Input: part model. Units: mm. Frame: model coordinates. Face numbers are marked on the shaded views. A direction names the side the tool comes from. Coordinates: 2 decimals unless noted, no trailing zeros. Order: outer loops, then holes, each group sorted by start corner. A loop starts at its lowest first (then second) coordinate and runs counter-clockwise, first axis right, second up. Notation, with made-up numbers: (5, 88) -> (51, 88) arc R8 ccw to (51, 95) -> close; hole circle Ø6 at (77, 84.25). An arc over 180 degrees is marked (long way). Answer as CSV lines item,"result".
from build123d import *

# Parameters (mm, degrees)
BOSS_EXTRUDE1_DEPTH      = 1.2
BOSS_EXTRUDE1_DEPTH_BACK = 1.2
SKETCH1_W                = 97
SKETCH1_H                = 71
SKETCH2_W                = 77
SKETCH2_H                = 51
CUT_EXTRUDE1_DEPTH       = 1.1
FILLET1_R                = 5
FILLET1_OF_MIRROR3_R     = 5
FILLET2_R                = 5


with BuildPart() as part:
    # Sketch1 → Boss-Extrude1 (new, two sides: drawn at the far end of the back side and taken through both)
    with BuildSketch(Plane(origin=(0, 0, 0), x_dir=(1, 0, 0), z_dir=(0, 1, 0)).offset(-BOSS_EXTRUDE1_DEPTH_BACK)):
        Rectangle(SKETCH1_W, SKETCH1_H)
    extrude(amount=BOSS_EXTRUDE1_DEPTH + BOSS_EXTRUDE1_DEPTH_BACK)

    # Sketch2 → Cut-Extrude1 (cut)
    with BuildSketch(Plane(origin=(0, 1.2, 0), x_dir=(1, 0, 0), z_dir=(0, 1, 0))):
        Rectangle(SKETCH2_W, SKETCH2_H)
    cut_extrude1 = extrude(amount=-CUT_EXTRUDE1_DEPTH, mode=Mode.SUBTRACT)

    # Fillet1
    fillet1_edges = [part.edges().sort_by_distance(p)[0] for p in [
        (38.5, 0.65, 25.5),
        (-38.5, 0.65, 25.5),
        (-38.5, 0.65, -25.5),
        (38.5, 0.65, -25.5),
    ]]
    fillet(fillet1_edges, radius=FILLET1_R)

    # Mirror3: Cut-Extrude1 across plane
    add(cut_extrude1.mirror(Plane.ZX), mode=Mode.SUBTRACT)

    # Fillet1 of Mirror3
    fillet1_of_mirror3_edges = [part.edges().sort_by_distance(p)[0] for p in [
        (38.5, -0.65, 25.5),
        (-38.5, -0.65, 25.5),
        (-38.5, -0.65, -25.5),
        (38.5, -0.65, -25.5),
    ]]
    fillet(fillet1_of_mirror3_edges, radius=FILLET1_OF_MIRROR3_R)

    # Fillet2
    fillet2_edges = [part.edges().sort_by_distance(p)[0] for p in [
        (48.5, 0, 35.5),
        (-48.5, 0, 35.5),
        (-48.5, 0, -35.5),
        (48.5, 0, -35.5),
    ]]
    fillet(fillet2_edges, radius=FILLET2_R)


solid = part.part
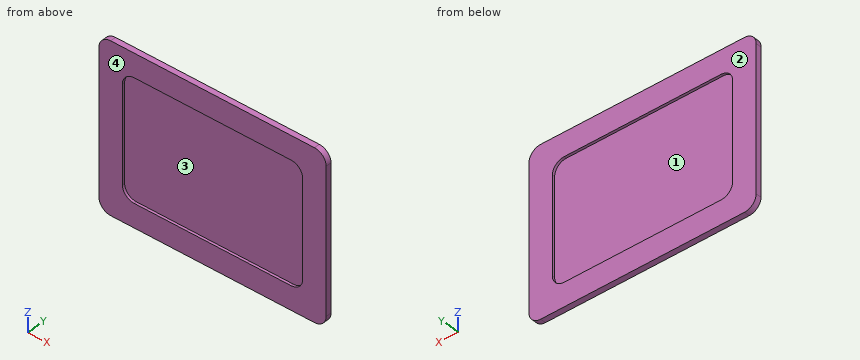
1. Cut plane A-A (y = -0.6). Return the cut outline in (x, z), plus the area to 3 significant figures.
Findings:
outline,"(-48.5, -30.5) arc R5 ccw to (-43.5, -35.5) -> (43.5, -35.5) arc R5 ccw to (48.5, -30.5) -> (48.5, 30.5) arc R5 ccw to (43.5, 35.5) -> (-43.5, 35.5) arc R5 ccw to (-48.5, 30.5) -> close; hole (-38.5, -20.5) arc R5 ccw to (-33.5, -25.5) -> (33.5, -25.5) arc R5 ccw to (38.5, -20.5) -> (38.5, 20.5) arc R5 ccw to (33.5, 25.5) -> (-33.5, 25.5) arc R5 ccw to (-38.5, 20.5) -> close"
area,"2,960 mm2"
2. Ray query, line 1 along X through (y, z) = (-1, 11); line 2 along Z through (x, y) = (-30.5, -0.6); line 3 along Y through (x, z) = (-35.5, -14.5). Return the intervals inside material, ascending.
Findings:
line 1,"x = -48.5 to -38.5, 38.5 to 48.5"
line 2,"z = -35.5 to -25.5, 25.5 to 35.5"
line 3,"y = -0.1 to 0.1"
3. Cut plane C-C (z = -7.5). Return the cut outline in (x, y).
Findings:
outline,"(-48.5, -1.2) -> (-38.5, -1.2) -> (-38.5, -0.1) -> (38.5, -0.1) -> (38.5, -1.2) -> (48.5, -1.2) -> (48.5, 1.2) -> (38.5, 1.2) -> (38.5, 0.1) -> (-38.5, 0.1) -> (-38.5, 1.2) -> (-48.5, 1.2) -> close"
4. Contact query for flat-ended pins moving along their axis: pin 1 (1 mm diameter, centred on x = -21, z = 4, fed in from +Y); pin 2 (4 mm diameter, centred on x = 17, z = 21.5, fed in from -Y). Output: stop coordinate, or through.
Findings:
pin 1,"stops at y = 0.1"
pin 2,"stops at y = -0.1"
5. Reachability of the marked faces 1 and 2 from +Z, -Z, +X, -X, +Y, -Y: full face, straight path, thin tool, end or side. Return the list, or none.
Findings:
face 1,"+Y"
face 2,"+Z, -Z, +X, -X, +Y"
6. Mould query, pull axis X, two halves, no side actions, for the marked faces 3 and 4. Classes: released by +X, released by -X, zero draft, split by the parting line, or undercut.
Findings:
face 3,"undercut"
face 4,"zero draft"
7. Cut plane B-B (x = 23). Return the cut outline in (y, z).
Findings:
outline,"(-1.2, -35.5) -> (1.2, -35.5) -> (1.2, -25.5) -> (0.1, -25.5) -> (0.1, 25.5) -> (1.2, 25.5) -> (1.2, 35.5) -> (-1.2, 35.5) -> (-1.2, 25.5) -> (-0.1, 25.5) -> (-0.1, -25.5) -> (-1.2, -25.5) -> close"
